```python
from build123d import *

# Parameters (mm, degrees)
EXTRUDE_1_DEPTH     = 2
EXTRUDE_2_DEPTH     = 5
SKETCH_3_W          = 2
SKETCH_3_H          = 1.9
SKETCH_3_H_2        = 2.9
EXTRUDE_3_DEPTH     = 3.2
SKETCH_4_W          = 3.15
SKETCH_4_H          = 1.9
SKETCH_4_H_2        = 2.9
SKETCH_4_W_2        = 3
EXTRUDE_4_DEPTH     = 3
SKETCH_6_W          = 3.15
SKETCH_6_H          = 2.9
SKETCH_6_H_2        = 1.9
EXTRUDE_5_DEPTH     = 0.7
EXTRUDE_6_DEPTH     = 1.9
EXTRUDE_7_DEPTH     = 2.9
EXTRUDE_8_DEPTH     = 2.9
EXTRUDE_9_DEPTH     = 2.9
FILLET_1_R          = 2
CUT_EXTRUDE_1_REACH = 61.364
SKETCH_12_W         = 4.7
SKETCH_12_H         = 9
EXTRUDE_10_DEPTH    = 0.8
CHAMFER_1_SIZE      = 1
CUT_EXTRUDE_2_DEPTH = 20
CUT_EXTRUDE_3_DEPTH = 4
FILLET_2_R          = 0.5


with BuildPart() as part:
    # 草图1 → 凸台-拉伸1 (new body)
    with BuildSketch(Plane.XY):
        with BuildLine():
            Line((-30, -35), (30, -35))
            ThreePointArc((30, -35), (33.535533906, -33.535533906), (35, -30))
            Line((35, -30), (35, 30))
            ThreePointArc((35, 30), (33.535533906, 33.535533906), (30, 35))
            Line((30, 35), (-30, 35))
            ThreePointArc((-30, 35), (-32.5, 34.330127019), (-34.330127019, 32.5))
            Line((-34.330127019, 32.5), (-35, 32.5))
            Line((-35, 32.5), (-35, 30))
            Line((-35, 30), (-35, -30))
            Line((-35, -30), (-35, -32.5))
            Line((-35, -32.5), (-34.330127019, -32.5))
            ThreePointArc((-34.330127019, -32.5), (-32.5, -34.330127019), (-30, -35))
        make_face()
    extrude(amount=EXTRUDE_1_DEPTH)

    # 草图2 → 凸台-拉伸2 (add)
    with BuildSketch(Plane(origin=(0, 0, 0), x_dir=(-1, 0, 0), z_dir=(0, 0, -1))):
        with BuildLine():
            Line((25.867224141, -32.95), (25.867224141, -29.95))
            ThreePointArc((25.867224141, -29.95), (23.117224141, -27.2), (20.367224141, -29.95))
            Line((20.367224141, -29.95), (20.367224141, -32.95))
            Line((20.367224141, -32.95), (25.867224141, -32.95))
        make_face()
        with BuildLine():
            Line((20.367224141, 32.95), (20.367224141, 29.95))
            ThreePointArc((20.367224141, 29.95), (23.117224141, 27.2), (25.867224141, 29.95))
            Line((25.867224141, 29.95), (25.867224141, 32.95))
            Line((25.867224141, 32.95), (20.367224141, 32.95))
        make_face()
        with BuildLine():
            Line((-23.357009719, -29.95), (-23.357009719, -32.95))
            Line((-23.357009719, -32.95), (-17.857009719, -32.95))
            Line((-17.857009719, -32.95), (-17.857009719, -29.95))
            ThreePointArc((-17.857009719, -29.95), (-20.607009719, -27.2), (-23.357009719, -29.95))
        make_face()
        with BuildLine():
            Line((-23.357009719, 32.95), (-17.857009719, 32.95))
            Line((-17.857009719, 32.95), (-17.857009719, 29.95))
            ThreePointArc((-17.857009719, 29.95), (-20.607009719, 27.2), (-23.357009719, 29.95))
            Line((-23.357009719, 29.95), (-23.357009719, 32.95))
        make_face()
    extrude(amount=EXTRUDE_2_DEPTH)

    # 草图3 → 凸台-拉伸3 (add)
    with BuildSketch(Plane(origin=(0, 0, 0), x_dir=(-1, 0, 0), z_dir=(0, 0, -1))):
        with Locations((31.9, -29)):
            Rectangle(SKETCH_3_W, SKETCH_3_H)
        with Locations((31.9, 21.5)):
            Rectangle(SKETCH_3_W, SKETCH_3_H_2)
        with Locations((-31.9, -5.5)):
            Rectangle(SKETCH_3_W, SKETCH_3_H_2)
        with Locations((-31.9, 11)):
            Rectangle(SKETCH_3_W, SKETCH_3_H_2)
    extrude(amount=EXTRUDE_3_DEPTH)

    # 草图4 → 凸台-拉伸4 (add)
    with BuildSketch(Plane(origin=(0, 0, -3.2), x_dir=(-1, 0, 0), z_dir=(0, 0, -1))):
        with Locations((32.475, -29)):
            Rectangle(SKETCH_4_W, SKETCH_4_H)
        with Locations((32.475, 21.5)):
            Rectangle(SKETCH_4_W, SKETCH_4_H_2)
        with Locations((-32.4, -5.5)):
            Rectangle(SKETCH_4_W_2, SKETCH_4_H_2)
        with Locations((-32.4, 11)):
            Rectangle(SKETCH_4_W_2, SKETCH_4_H_2)
    extrude(amount=EXTRUDE_4_DEPTH)

    # 草图6 → 凸台-拉伸5 (add)
    with BuildSketch(Plane(origin=(0, 0, -6.2), x_dir=(-1, 0, 0), z_dir=(0, 0, -1))):
        with Locations((32.475, 21.5)):
            Rectangle(SKETCH_6_W, SKETCH_6_H)
        with Locations((32.475, -29)):
            Rectangle(SKETCH_6_W, SKETCH_6_H_2)
    extrude(amount=EXTRUDE_5_DEPTH)

    # 草图7 → 凸台-拉伸6 (add)
    with BuildSketch(Plane.XZ.offset(29.95)):
        Polygon((-30.9, -6.9), (-26.916283143, 0), (-30.9, 0), align=None)
    extrude(amount=-EXTRUDE_6_DEPTH)

    # 草图8 → 凸台-拉伸7 (add)
    with BuildSketch(Plane(origin=(0, 22.95, 0), x_dir=(1, 0, 0), z_dir=(0, 1, 0))):
        Polygon((-30.9, 6.9), (-26.916283143, 0), (-30.9, 0), align=None)
    extrude(amount=-EXTRUDE_7_DEPTH)

    # 草图9 → 凸台-拉伸8 (add)
    with BuildSketch(Plane(origin=(0, 12.45, 0), x_dir=(1, 0, 0), z_dir=(0, 1, 0))):
        Polygon((30.9, 6.2), (27.320428331, 0), (30.9, 0), align=None)
    extrude(amount=-EXTRUDE_8_DEPTH)

    # 草图10 → 凸台-拉伸9 (add)
    with BuildSketch(Plane.XZ.offset(6.95)):
        Polygon((30.9, -6.2), (27.320428331, 0), (30.9, 0), align=None)
    extrude(amount=-EXTRUDE_9_DEPTH)

    # 圆角1
    fillet_1_edges = [part.edges().sort_by_distance(p)[0] for p in [
        (-29.908141571, 22.95, 0),
        (-29.908141571, 20.05, 0),
        (30.110214166, -6.95, 0),
        (30.110214166, 12.45, 0),
        (-29.908141571, -28.05, 0),
        (-29.908141571, -29.95, 0),
    ]]
    fillet(fillet_1_edges, radius=FILLET_1_R)

    # 切除-拉伸1: up to this face of the body (flat: up to its plane)
    cut_extrude_1_end = Plane(part.part.faces().sort_by_distance((31.614518318, -6.95, -3.993006547))[0])
    # 草图11 → 切除-拉伸1 (cut, up to the picked face)
    with BuildSketch(Plane(origin=(0, 12.45, 0), x_dir=(1, 0, 0), z_dir=(0, 1, 0)), mode=Mode.PRIVATE) as cut_extrude_1_sk1:
        Polygon((33.4, 3.2), (33.9, 3.7), (33.9, 3.2), align=None)
    cut_extrude_1_tool1 = split(extrude(cut_extrude_1_sk1.sketch, amount=-CUT_EXTRUDE_1_REACH, mode=Mode.PRIVATE), bisect_by=cut_extrude_1_end, keep=Keep.BOTH, mode=Mode.PRIVATE)
    add(cut_extrude_1_tool1.solids().sort_by(Axis((33.733333, 12.45, -3.366667), (0, -1, 0)))[0], mode=Mode.SUBTRACT)

    # 草图12 → 凸台-拉伸10 (add)
    with BuildSketch(Plane(origin=(0, 0, 0), x_dir=(-1, 0, 0), z_dir=(0, 0, -1))):
        with Locations((-29.65, 2.733632703)):
            Rectangle(SKETCH_12_W, SKETCH_12_H)
    extrude(amount=EXTRUDE_10_DEPTH)

    # 倒角1
    chamfer_1_edges = [part.edges().sort_by_distance(p)[0] for p in [
        (33.9, -5.5, -6.2),
        (33.9, 11, -6.2),
    ]]
    chamfer(chamfer_1_edges, length=CHAMFER_1_SIZE)

    # 草图13 → 切除-拉伸2 (cut)
    with BuildSketch(Plane.XZ.offset(6.95)):
        Polygon((32.9, -3.2), (33.4, -3.7), (33.4, -5.430067518), (32.9, -6.2), (33.9, -5.2), (33.9, -3.7), (33.4, -3.2), align=None)
    extrude(amount=-CUT_EXTRUDE_2_DEPTH, mode=Mode.SUBTRACT)

    # 草图14 → 切除-拉伸3 (cut)
    with BuildSketch(Plane(origin=(0, 0, -6.2), x_dir=(-1, 0, 0), z_dir=(0, 0, -1))):
        Polygon((-33.4, 12.15), (-31.9, 12.45), (-33.4, 12.45), align=None)
        Polygon((-33.4, 9.55), (-33.4, 9.85), (-31.9, 9.55), align=None)
        Polygon((-33.4, -4.05), (-33.4, -4.35), (-31.9, -4.05), align=None)
        Polygon((-33.4, -6.95), (-31.9, -6.95), (-33.4, -6.65), align=None)
    extrude(amount=-CUT_EXTRUDE_3_DEPTH, mode=Mode.SUBTRACT)

    # 圆角2
    # the kernel refuses this fillet: 0.5 mm, written as the material it adds along each edge
    with BuildSketch(Plane(origin=(34.125725845, 9.995145169, -2.2), x_dir=(0, 0, -1), z_dir=(-0.9805806756909201, -0.1961161351381845, 0))) as fillet_2_piece_1_section:
        with BuildLine():
            CenterArc((FILLET_2_R, FILLET_2_R), FILLET_2_R, 180, 90)
            Line((0, FILLET_2_R), (0, 0))
            Line((0, 0), (FILLET_2_R, 0))
        make_face()
    fillet_2_piece_1 = extrude(amount=3.519803903, mode=Mode.PRIVATE)
    fillet_2_piece_1 = split(fillet_2_piece_1, bisect_by=Plane(origin=(32.9, 9.624038043, -2.351425579), z_dir=(-1, 0, 0)), keep=Keep.TOP, mode=Mode.PRIVATE)
    fillet_2_piece_1 = split(fillet_2_piece_1, bisect_by=Plane(origin=(32.529809776, 9.55, -2.351425579), z_dir=(0, 1, 0)), keep=Keep.TOP, mode=Mode.PRIVATE)
    add(fillet_2_piece_1)
    with BuildSketch(Plane(origin=(34.125725845, 12.004854831, -2.2), x_dir=(0.1961161351381845, 0.9805806756909201, 0), z_dir=(-0.9805806756909201, 0.1961161351381845, 0))) as fillet_2_piece_2_section:
        with BuildLine():
            CenterArc((FILLET_2_R, FILLET_2_R), FILLET_2_R, 180, 90)
            Line((0, FILLET_2_R), (0, 0))
            Line((0, 0), (FILLET_2_R, 0))
        make_face()
    fillet_2_piece_2 = extrude(amount=3.519803903, mode=Mode.PRIVATE)
    fillet_2_piece_2 = split(fillet_2_piece_2, bisect_by=Plane(origin=(32.9, 12.375961957, -2.351425579), z_dir=(-1, 0, 0)), keep=Keep.TOP, mode=Mode.PRIVATE)
    fillet_2_piece_2 = split(fillet_2_piece_2, bisect_by=Plane(origin=(32.529809778, 12.45, -2.351425579), z_dir=(0, -1, 0)), keep=Keep.TOP, mode=Mode.PRIVATE)
    add(fillet_2_piece_2)
    with BuildSketch(Plane(origin=(34.125725845, -4.495145169, -2.2), x_dir=(0, 0, -1), z_dir=(-0.9805806756909202, 0.1961161351381839, 0))) as fillet_2_piece_3_section:
        with BuildLine():
            CenterArc((FILLET_2_R, -FILLET_2_R), FILLET_2_R, 90, 90)
            Line((0, -FILLET_2_R), (0, 0))
            Line((0, 0), (FILLET_2_R, 0))
        make_face()
    fillet_2_piece_3 = extrude(amount=3.519803903, mode=Mode.PRIVATE)
    fillet_2_piece_3 = split(fillet_2_piece_3, bisect_by=Plane(origin=(32.529809776, -4.05, -2.351425579), z_dir=(0, -1, 0)), keep=Keep.TOP, mode=Mode.PRIVATE)
    fillet_2_piece_3 = split(fillet_2_piece_3, bisect_by=Plane(origin=(32.9, -4.124038043, -2.351425579), z_dir=(-1, 0, 0)), keep=Keep.TOP, mode=Mode.PRIVATE)
    add(fillet_2_piece_3)
    with BuildSketch(Plane(origin=(30.674274155, -7.195145169, -2.2), x_dir=(0, 0, -1), z_dir=(0.9805806756909202, 0.1961161351381839, 0))) as fillet_2_piece_4_section:
        with BuildLine():
            CenterArc((FILLET_2_R, -FILLET_2_R), FILLET_2_R, 90, 90)
            Line((0, -FILLET_2_R), (0, 0))
            Line((0, 0), (FILLET_2_R, 0))
        make_face()
    fillet_2_piece_4 = extrude(amount=3.519803903, mode=Mode.PRIVATE)
    fillet_2_piece_4 = split(fillet_2_piece_4, bisect_by=Plane(origin=(32.9, -6.875961957, -2.351425579), z_dir=(-1, 0, 0)), keep=Keep.TOP, mode=Mode.PRIVATE)
    fillet_2_piece_4 = split(fillet_2_piece_4, bisect_by=Plane(origin=(32.529809776, -6.95, -2.351425579), z_dir=(0, 1, 0)), keep=Keep.TOP, mode=Mode.PRIVATE)
    add(fillet_2_piece_4)


solid = part.part
```
Check sheet for the modelled part. Datum: model origin and axes. Units: mm. A direction names the side the tool comes from. Round coordinates to 2 decimals unless told otherwise and drop trailing zeros. Order: outer loops, then holes, each group sorted by start corner. A loop starts at its lowest first (then second) coordinate and runs counter-clockwise, first axis right, second up. Notation, with made-up numbers: (15.25, 29.25) -> (24.25, 29.25) arc R37 cw to (24.25, 68.25) -> close; hole circle Ø10 at (-29, 48.5). An arc over 180 degrees is marked (long way). One line per item, written item: value. Start each with the question number.
Q1. Cross-section at B-B (x = 19). Record the boundary of the cut face in (y, z), and give its area (3 significant figures).
Q2. Gauge pin test, flat ends, axial feed: pin 1 Ø3.5 at (x, z) = (30.5, -4) entering from -Y; pin 2 Ø4 at (x, z) = (21.5, -3) entering from -Y; pin 3 Ø2.5 at (y, z) = (-31, -2.5) entering from +X. Record the tip position at first contact, or that the pin passes through.
Q3. Mould release check, pull along X, two halves, no side actions. Record for faces 5 (the face through (29.135, -5.445, -3.143)), 6 (the face through (-20.367, -31, -2)), 7 (the face through (0, 0, 2)), 8 (the face through (17.857, 31, -2)): pulls with the +X half, pulls with the -X half, needs draft (parallel to the pull), parting line crosses it, or undercut.
Q4. Cross-section at C-C (x = 1). Record the boundary of the cut face in (y, z), and give its area (3 significant figures).
Q5. Thickness scan on line 1 (X direction, y = 31, z = -3.5); line 2 (Y direction, x = -30.5, z = -6); line 3 (Z direction, x = -22.5, y = -22). Record the ranges inside material, lowest first.
Q6. Set-up check for faces 1 (the face through (-23, -30, -5)), 2 (the face through (-23.1, 27.2, -2.5)), 3 (the face through (32.9, 11, -2)), 4 (the face through (-34.05, 21, -5)): record each of +Z, -Z, +X, -X, +Y, -Y from which the full face is reachable in a straight line by a thin tool's end or side.
Q7. Cross-section at A-A (y = 3.5). Record the boundary of the cut face in (x, z).
Completed:
1. outline: (-35, 0) -> (-32.95, 0) -> (-32.95, -5) -> (-27.72, -5) -> (-27.72, 0) -> (27.72, 0) -> (27.72, -5) -> (32.95, -5) -> (32.95, 0) -> (35, 0) -> (35, 2) -> (-35, 2) -> close
1. area: 192 mm²
2. pin 1: stops at y = -6.95
2. pin 2: stops at y = -32.95
2. pin 3: stops at x = 23.36
3. face 5: pulls with the -X half
3. face 6: undercut
3. face 7: needs draft
3. face 8: undercut
4. outline: (-35, 0) -> (35, 0) -> (35, 2) -> (-35, 2) -> close
4. area: 140 mm²
5. line 1: x = -25.87 to -20.37, 17.86 to 23.36
5. line 2: y = -29.95 to -28.05, 20.05 to 22.95
5. line 3: z = 0 to 2
6. face 1: -Z, +X, +Y, -Y
6. face 2: -Z
6. face 3: +X, +Y, -Y
6. face 4: -Z, -X, +Y, -Y
7. outline: (-35, 0) -> (27.3, 0) -> (27.3, -0.8) -> (32, -0.8) -> (32, 0) -> (35, 0) -> (35, 2) -> (-35, 2) -> close
